Can you work these out from the model? Positions are in its coordinate system, mm. Face numbers are marked on the shaded views. A direction names the side the tool comes from. Round coordinates to 2 decimals unless told otherwise and drop trailing zeros. Order: outer loops, then holes, each group sorted by start corner. A loop starts at its lowest first (then second) coordinate and runs counter-clockwise, first axis right, second up.
Q1. If we section it at A-A (z = 30): Please give me the cut outline in (x, y).
Q2. Will these pins go through, and if not, where does the flat tip stop? P1, Ø6, axis at y = 15, z = 27, coming from the -X side; P2, Ø1, axis at x = -8.5, y = -2.5, coming from the -Z side; P3, Ø4, axis at x = -22, y = -1, coming from the +Z side; P4, Ø2, axis at x = -28, z = 12, coming from the +Y side.
Q3. We'd pull the mould along X, two halves only. Please class the marked faces 1, 2 and 3: pulls with the +X half, pulls with the -X half, needs draft (parallel to the pull), parting line crosses it, or undercut.
Q4. If I drill on line 1 (Y direction, x = -32, z = 31.5); line 2 (X direction, y = 11.5, z = 7); line 3 (X direction, y = 35, z = 12), over which ranges is the centre line in solid material (lowest first)?
Q5. For the marked faces 4, 5, 6 and 7, which set-ups out of +Z, -Z, +X, -X, +Y, -Y let a thin tool reach every point of the face, with its end or its side?
Q6. If we section it at D-D (y = 24): Please give me the cut outline in (x, z), plus the area to 3 significant figures.
Q7. If we section it at B-B (y = 7.5): Please give me the cut outline in (x, z), plus the area to 3 significant figures.
from build123d import *

# Parameters (mm, degrees)
SKETCH_W        = 76.142136
SKETCH_H        = 76.142136
PAD_DEPTH       = 25.4
SKETCH001_W     = 20
SKETCH001_H     = 20
PAD001_DEPTH    = 25.4
SKETCH002_W     = 65
SKETCH002_H     = 65
POCKET_DEPTH    = 8.35
SKETCH003_R     = 2.1463
POCKET001_DEPTH = 10


with BuildPart() as part:
    # Sketch → Pad (new body)
    with BuildSketch(Plane.XY):
        Rectangle(SKETCH_W, SKETCH_H)
    extrude(amount=PAD_DEPTH)

    # Sketch001 (on Face6 of Pad) → Pad001 (join)
    with BuildSketch(Plane.XY.offset(25.4)):
        with Locations((-28.071068, 28.071068)):
            Rectangle(SKETCH001_W, SKETCH001_H)
        with Locations((28.071068, 28.071068)):
            Rectangle(SKETCH001_W, SKETCH001_H)
        with Locations((28.071068, -28.071068)):
            Rectangle(SKETCH001_W, SKETCH001_H)
        with Locations((-28.071068, -28.071068)):
            Rectangle(SKETCH001_W, SKETCH001_H)
    extrude(amount=PAD001_DEPTH)

    # Sketch002 (on Face4 of Pad001) → Pocket (cut)
    with BuildSketch(Plane(origin=(0, 0, 0), x_dir=(1, 0, 0), z_dir=(0, 0, -1))):
        Rectangle(SKETCH002_W, SKETCH002_H)
    extrude(amount=-POCKET_DEPTH, mode=Mode.SUBTRACT)

    # Sketch003 (on Face1 of Pocket) → Pocket001 (cut)
    with BuildSketch(Plane(origin=(0, 38.071068, 0), x_dir=(-1, 0, 0), z_dir=(0, 1, 0))):
        with Locations((-28.071068, 12.7)):
            Circle(SKETCH003_R)
        with Locations((28.071068, 12.7)):
            Circle(SKETCH003_R)
    extrude(amount=-POCKET001_DEPTH, mode=Mode.SUBTRACT)


solid = part.part
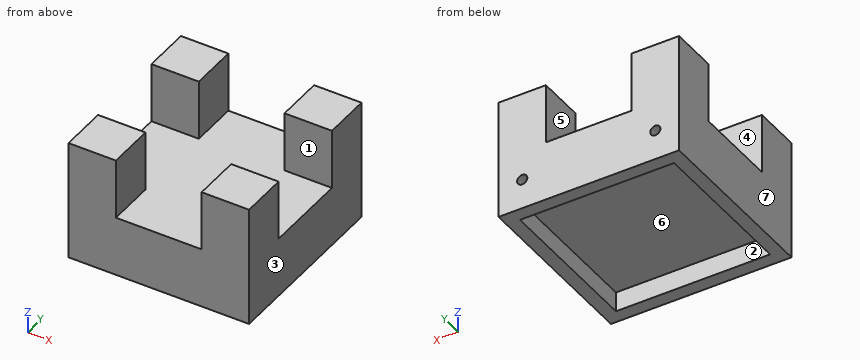
Solution:
1. outline: (-38.07, -38.07) - (-18.07, -38.07) - (-18.07, -18.07) - (-38.07, -18.07) - close; (-38.07, 18.07) - (-18.07, 18.07) - (-18.07, 38.07) - (-38.07, 38.07) - close; (18.07, -38.07) - (38.07, -38.07) - (38.07, -18.07) - (18.07, -18.07) - close; (18.07, 18.07) - (38.07, 18.07) - (38.07, 38.07) - (18.07, 38.07) - close
2. P1: stops at x = -38.07
2. P2: stops at z = 8.35
2. P3: stops at z = 25.4
2. P4: stops at y = 28.07
3. face 1: needs draft
3. face 2: undercut
3. face 3: pulls with the +X half
4. line 1: y = -38.07 to -18.07, 18.07 to 38.07
4. line 2: x = -38.07 to -32.5, 32.5 to 38.07
4. line 3: x = -38.07 to -30.1, -26.04 to 26.04, 30.1 to 38.07
5. face 4: +Z, +X, -X
5. face 5: +Z, +Y, -Y
5. face 6: -Z
5. face 7: +Z, -Z, -X, +Y, -Y
6. outline: (-38.07, 0) - (-32.5, 0) - (-32.5, 8.35) - (32.5, 8.35) - (32.5, 0) - (38.07, 0) - (38.07, 50.8) - (18.07, 50.8) - (18.07, 25.4) - (-18.07, 25.4) - (-18.07, 50.8) - (-38.07, 50.8) - close
6. area: 2,410 mm2
7. outline: (-38.07, 0) - (-32.5, 0) - (-32.5, 8.35) - (32.5, 8.35) - (32.5, 0) - (38.07, 0) - (38.07, 25.4) - (-38.07, 25.4) - close
7. area: 1,390 mm2
